```python
from build123d import *

# Parameters (mm, degrees)
SKETCH_R   = 2.15
SKETCH_R_2 = 5
PAD_DEPTH  = 3


with BuildPart() as part:
    # Sketch → Pad (new body)
    with BuildSketch(Plane.XY):
        with BuildLine():
            Line((36.7, 0.5), (85, 0.5))
            ThreePointArc((85, 0.5), (86.06066, 0.93934), (86.5, 2))
            Line((86.5, 2), (86.5, 37.1))
            ThreePointArc((88, 38.6), (86.93934, 38.16066), (86.5, 37.1))
            Line((88, 38.6), (123.1, 38.6))
            ThreePointArc((123.1, 38.6), (124.16066, 39.03934), (124.6, 40.1))
            Line((124.6, 40.1), (124.6, 100.6))
            ThreePointArc((124.6, 100.6), (124.16066, 101.66066), (123.1, 102.1))
            Line((123.1, 102.1), (85, 102.1))
            Line((85, 102.1), (37.720623, 102.1))
            ThreePointArc((37.720623, 102.1), (36.876806, 101.84015), (36.325343, 101.150631))
            Line((3.720746, 18.531652), (36.325343, 101.150631))
            ThreePointArc((0, 16), (2.250179, 16.692932), (3.720746, 18.531652))
            ThreePointArc((0, 16), (-12.263768, -10.276186), (15.753095, -2.8))
            ThreePointArc((19.691369, 0.5), (17.122322, -0.434058), (15.753095, -2.8))
            Line((36.7, 0.5), (19.691369, 0.5))
        make_face()
        with Locations((-8, 8)):
            Circle(SKETCH_R, mode=Mode.SUBTRACT)
        with Locations((8, 8)):
            Circle(SKETCH_R, mode=Mode.SUBTRACT)
        with Locations((-8, -8)):
            Circle(SKETCH_R, mode=Mode.SUBTRACT)
        with Locations((8, -8)):
            Circle(SKETCH_R, mode=Mode.SUBTRACT)
        Circle(SKETCH_R_2, mode=Mode.SUBTRACT)
    extrude(amount=PAD_DEPTH)


solid = part.part
```
Build history of the part. All positions in model axes, mm. A direction names the side the tool comes from. Coordinates: 2 decimals unless noted, no trailing zeros. Order: outer loops, then holes, each group sorted by start corner. A loop starts at its lowest first (then second) coordinate and runs counter-clockwise, first axis right, second up. Notation, with made-up numbers: M 86.25,30 L 120.25,30 A32 cw 120.25,65 Z; hole C -38.75,88.25 d8. An arc over 180 degrees is marked long. One line per question, with ' | ' between items. Start each with the question number.
1. Cut at A-A (x = 8). Write the cut outline in (y, z), plus the area to 3 significant figures.
2. Flat gauge pins, fed straight in: P1, Ø1.5, axis at x = 106, z = 2, coming from the -Y side; P2, Ø0.9, axis at x = 47, z = 1, coming from the -Y side. Where does each tip first touch, or does it go through?
3. Tool access for faces 1 (the face through (52, 0.5, 1)), 2 (the face through (69, 44, 3)): list every direction of +Z, -Z, +X, -X, +Y, -Y with a clear straight run to the whole face (end or side of a thin tool).
4. Mould opens along Y. For faces 3 (the face through (81, 102.1, 1)), 4 (the face through (17.15, -0.41, 1.48)), 5 (the face through (-8.28, -5.87, 1.48)), 6 (the face through (124.6, 70, 1)) say: +Y half, -Y half, draft (parallel to the pull), parting line (faces both ways), or undercut.
5. Cut at C-C (z = 2.05). Write the cut outline in (x, y), plus the area to 3 significant figures.
6. Wall check: line 1 along Y through (x, z) = (-0.5, 0.4); line 2 along Y through (x, z) = (-8, 1.9); line 3 along X through (y, z) = (9, 2.6). Give the ranges that are in metal, low to high. Write a range as [from, to].
7. Cut at B-B (y = 8). Write the cut outline in (x, z), plus the area to 3 significant figures.
8. Cut at D-D (x = 68.5). Write the cut outline in (y, z).
The answers:
1) outline: M -13.86,0 L -10.15,0 L -10.15,3 L -13.86,3 Z; M -5.85,0 L 5.85,0 L 5.85,3 L -5.85,3 Z; M 10.15,0 L 29.38,0 L 29.38,3 L 10.15,3 Z | area: 104 mm2
2) P1: stops at y = 38.6 | P2: stops at y = 0.5
3) face 1: +Z, -Z, +X, -Y | face 2: +Z, +X, -X, +Y, -Y
4) face 3: +Y half | face 4: -Y half | face 5: undercut | face 6: draft
5) outline: M 0,16 A16 ccw long 15.75,-2.8 A4 cw 19.69,0.5 L 85,0.5 A1.5 ccw 86.5,2 L 86.5,37.1 A1.5 cw 88,38.6 L 123.1,38.6 A1.5 ccw 124.6,40.1 L 124.6,100.6 A1.5 ccw 123.1,102.1 L 37.72,102.1 A1.5 ccw 36.33,101.15 L 3.72,18.53 A4 cw Z; hole C -8,-8 d4.3; hole C -8,8 d4.3; hole C 0,0 d10; hole C 8,-8 d4.3; hole C 8,8 d4.3 | area: 9,990 mm2
6) line 1: y = [-15.99, -4.97], [4.97, 15.99] | line 2: y = [-13.86, -10.15], [-5.85, 5.85], [10.15, 13.86] | line 3: x = [-13.23, -9.9], [-6.1, 6.1], [9.9, 86.5]
7) outline: M -13.86,0 L -10.15,0 L -10.15,3 L -13.86,3 Z; M -5.85,0 L 5.85,0 L 5.85,3 L -5.85,3 Z; M 10.15,0 L 86.5,0 L 86.5,3 L 10.15,3 Z | area: 275 mm2
8) outline: M 0.5,0 L 102.1,0 L 102.1,3 L 0.5,3 Z
